Input: part model. Units: mm. Frame: model coordinates. Face numbers are marked on the shaded views. A direction names the side the tool comes from. Give positions to 0.01 mm unless a question says otherwise; leave off trailing zeros. Loops run counter-clockwise (first coordinate to the right, second up) from the corner with the lowest first, then second, coordinate; pieces in that order, holes last. Notation, with made-up numbers: (15.25, 66) -> (32.25, 66) arc R14 cw to (32.25, 80) -> close; hole circle Ø11 at (-38.5, 45). An arc over 180 degrees is marked (long way). Use CSV: the item, a comma, the result in double quotes.
```python
from build123d import *

# Parameters (mm, degrees)
SKETCH2_W           = 34.2
SKETCH2_H           = 23.2
SKETCH2_W_2         = 24.2
SKETCH2_H_2         = 13.2
BOSS_EXTRUDE1_DEPTH = 21
SKETCH2_2_W         = 34.2
SKETCH2_2_H         = 23.2
SKETCH2_2_W_2       = 24.2
SKETCH2_2_H_2       = 13.2
BOSS_EXTRUDE2_DEPTH = 8
BOSS_EXTRUDE3_DEPTH = 23.2
SKETCH3_R           = 1.6
CUT_EXTRUDE1_DEPTH  = 39.309920386
FILLET1_R           = 2
SKETCH5_W           = 5
SKETCH5_H           = 7
CUT_EXTRUDE2_DEPTH  = 19
SKETCH6_R           = 1.25
CUT_EXTRUDE3_DEPTH  = 6


with BuildPart() as part:
    # Sketch2 → Boss-Extrude1 (new body)
    with BuildSketch(Plane.XY):
        Rectangle(SKETCH2_W, SKETCH2_H)
        Rectangle(SKETCH2_W_2, SKETCH2_H_2, mode=Mode.SUBTRACT)
    extrude(amount=BOSS_EXTRUDE1_DEPTH)

    # Sketch2<2> → Boss-Extrude2 (add)
    # profile 1 of 2: a face of its own
    with BuildSketch(Plane.XY):
        Rectangle(SKETCH2_2_W, SKETCH2_2_H)
        Rectangle(SKETCH2_2_W_2, SKETCH2_2_H_2, mode=Mode.SUBTRACT)
    # profile 2 of 2: a face of its own
    with BuildSketch(Plane.XY):
        Rectangle(SKETCH2_2_W_2, SKETCH2_2_H_2)
    extrude(amount=-BOSS_EXTRUDE2_DEPTH)

    # Sketch4 → Boss-Extrude3 (add)
    with BuildSketch(Plane.XZ.offset(11.6)):
        Polygon((12.1, 0), (-12.1, 0), (-22.1, 0), (-22.1, -8), (-17.1, -8), (17.1, -8), (22.1, -8), (22.1, 0), align=None)
    extrude(amount=-BOSS_EXTRUDE3_DEPTH)

    # Sketch3 → Cut-Extrude1 (cut, through all)
    with BuildSketch(Plane.XZ.offset(11.6)):
        with Locations(Location((-15, -4, 0), (0, 0, 270))):
            Circle(SKETCH3_R)
        with Locations(Location((15, -4, 0), (0, 0, 270))):
            Circle(SKETCH3_R)
    extrude(amount=-CUT_EXTRUDE1_DEPTH, mode=Mode.SUBTRACT)

    # Fillet1
    fillet1_edges = [part.edges().sort_by_distance(p)[0] for p in [
        (0, -11.6, -8),
        (0, 11.6, -8),
        (-17.1, 0, 0),
        (22.1, 0, -8),
        (17.1, 0, 0),
        (-22.1, 0, 0),
        (19.6, -11.6, 0),
        (22.1, -11.6, -4),
        (-19.6, -11.6, 0),
        (-22.1, -11.6, -4),
        (19.6, 11.6, 0),
        (22.1, 11.6, -4),
        (-19.6, 11.6, 0),
        (-22.1, 11.6, -4),
        (22.1, 0, 0),
        (-22.1, 0, -8),
        (-17.1, -11.6, 10.5),
        (-17.1, 11.6, 10.5),
        (17.1, 11.6, 10.5),
        (17.1, -11.6, 10.5),
    ]]
    fillet(fillet1_edges, radius=FILLET1_R)

    # Sketch5 → Cut-Extrude2 (cut)
    with BuildSketch(Plane.XY.offset(21)):
        with Locations((-14.6, 0)):
            Rectangle(SKETCH5_W, SKETCH5_H)
    extrude(amount=-CUT_EXTRUDE2_DEPTH, mode=Mode.SUBTRACT)

    # Sketch6 → Cut-Extrude3 (cut)
    with BuildSketch(Plane.XY.offset(21)):
        with Locations((14.6, 3.5)):
            Circle(SKETCH6_R)
        with Locations(Location((14.6, -3.5, 0), (0, 0, 180))):
            Circle(SKETCH6_R)
    extrude(amount=-CUT_EXTRUDE3_DEPTH, mode=Mode.SUBTRACT)


solid = part.part
```
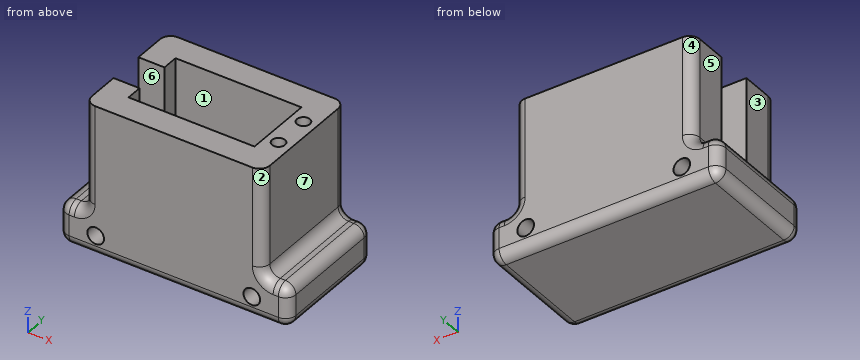
1) Section query A-A (z = 18.5). Return loops of the section in (x, y), then the cut area to 3 significant figures.
From the geometry:
outline,"(-17.1, -9.6) arc R2 ccw to (-15.1, -11.6) -> (15.1, -11.6) arc R2 ccw to (17.1, -9.6) -> (17.1, 9.6) arc R2 ccw to (15.1, 11.6) -> (-15.1, 11.6) arc R2 ccw to (-17.1, 9.6) -> (-17.1, 3.5) -> (-12.1, 3.5) -> (-12.1, 6.6) -> (12.1, 6.6) -> (12.1, -6.6) -> (-12.1, -6.6) -> (-12.1, -3.5) -> (-17.1, -3.5) -> close; hole circle Ø2.5 at (14.6, -3.5); hole circle Ø2.5 at (14.6, 3.5)"
area,"426 mm^2"
2) Section query B-B (x = -6). Return loops of the section in (y, z), then the cut area to 3 significant figures.
From the geometry:
outline,"(-11.6, -6) arc R2 ccw to (-9.6, -8) -> (9.6, -8) arc R2 ccw to (11.6, -6) -> (11.6, 21) -> (6.6, 21) -> (6.6, 0) -> (-6.6, 0) -> (-6.6, 21) -> (-11.6, 21) -> close"
area,"394 mm^2"
3) Ray query, line 1 (X direction, y = 4.5, z = -4); line 2 (Y direction, x = 14.6, z = 19.75); line 3 (Y direction, x = 5, z = 2.25). Return the intervals inside material, ascending.
From the geometry:
line 1,"x = -22.1 to -16.6, -13.4 to 13.4, 16.6 to 22.1"
line 2,"y = -11.6 to -4.75, -2.25 to 2.25, 4.75 to 11.6"
line 3,"y = -11.6 to -6.6, 6.6 to 11.6"
4) Mould query, pull axis X, two halves, no side actions, for the marked faces 1, 2 and 3. Classes: pulls with the +X half, pulls with the -X half, needs draft (parallel to the pull), parting line crosses it, or undercut.
From the geometry:
face 1,"undercut"
face 2,"pulls with the +X half"
face 3,"pulls with the -X half"
5) Section query C-C (y = -7.5). Return loops of the section in (x, z).
From the geometry:
outline,"(-22.1, -6) arc R2 ccw to (-20.1, -8) -> (20.1, -8) arc R2 ccw to (22.1, -6) -> (22.1, -2) arc R2 ccw to (20.1, 0) -> (19.1, 0) arc R2 cw to (17.1, 2) -> (17.1, 21) -> (-17.1, 21) -> (-17.1, 2) arc R2 cw to (-19.1, 0) -> (-20.1, 0) arc R2 ccw to (-22.1, -2) -> close; hole circle Ø3.2 at (-15, -4); hole circle Ø3.2 at (15, -4)"
6) Reachability of the marked faces 4, 5, 6 and 7 from +Z, -Z, +X, -X, +Y, -Y: full face, straight path, thin tool, end or side. Return the list, or none.
From the geometry:
face 4,"+Z, -X, +Y"
face 5,"+Z, -X, +Y, -Y"
face 6,"+Z, -X"
face 7,"+Z, +X, +Y, -Y"
7) Section query D-D (y = -3). Return loops of the section in (x, z).
From the geometry:
outline,"(-22.1, -6) arc R2 ccw to (-20.1, -8) -> (20.1, -8) arc R2 ccw to (22.1, -6) -> (22.1, -2) arc R2 ccw to (20.1, 0) -> (19.1, 0) arc R2 cw to (17.1, 2) -> (17.1, 21) -> (15.75, 21) -> (15.75, 15) -> (13.45, 15) -> (13.45, 21) -> (12.1, 21) -> (12.1, 0) -> (-12.1, 0) -> (-12.1, 2) -> (-17.1, 2) arc R2 cw to (-19.1, 0) -> (-20.1, 0) arc R2 ccw to (-22.1, -2) -> close; hole circle Ø3.2 at (-15, -4); hole circle Ø3.2 at (15, -4)"
8) Contact query for flat-ended pins moving along their axis: pin 1 (5 mm diameter, centred on y = 8, z = 5.5, fed in from -X); pin 2 (4 mm diameter, centred on x = 2.5, y = -2, fed in from +Z); pin 3 (9.5 mm diameter, centred on y = -3, z = 7, fed in from +X); pin 4 (1.5 mm diameter, centred on x = -15.5, z = 13.5, fed in from +Y). Output: stop coordinate, or through.
From the geometry:
pin 1,"stops at x = -17.1"
pin 2,"stops at z = 0"
pin 3,"stops at x = 17.1"
pin 4,"stops at y = 11.6"
